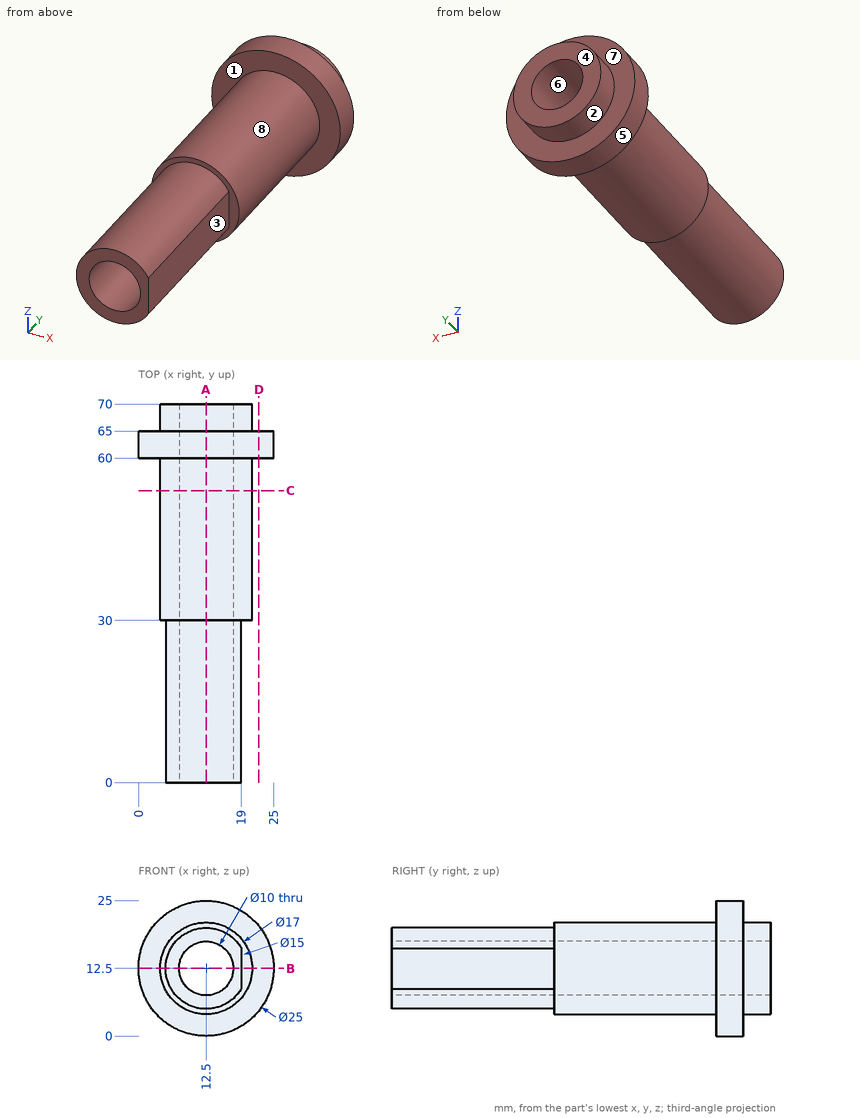
Here's the drawing with two shaded views (mm, measured from the low corner). I have some questions. A direction names the side the tool comes from. Coordinates: 2 decimals unless noted, no trailing zeros. Order: outer loops, then holes, each group sorted by start corner. A loop starts at its lowest first (then second) coordinate and runs counter-clockwise, first axis right, second up.
Item 1: I'm going to push flat-ended pins straight in: pin 1 Ø5 at (y, z) = (11.5, 7.5) entering from +X; pin 2 Ø8 at (x, y) = (21.5, 19.5) entering from -Z; pin 3 Ø1 at (x, y) = (7, 16) entering from +Z. Where does each tip first touch, or does it pass through?
Response values:
pin 1: stops at x = 19
pin 2: stops at z = 6.91
pin 3: stops at z = 18.09
Item 2: If we section it at B-B, the plane z = 12.5: List the corners of the cut face in (x, y) for me.
Response values:
outline: (0, 60) - (4, 60) - (4, 30) - (5, 30) - (5, 0) - (7.5, 0) - (7.5, 70) - (4, 70) - (4, 65) - (0, 65) - close; (17.5, 0) - (19, 0) - (19, 30) - (21, 30) - (21, 60) - (25, 60) - (25, 65) - (21, 65) - (21, 70) - (17.5, 70) - close
Item 3: If we section it at A-A, the plane x = 12.5: List the corners of the cut face in (y, z) for me.
Response values:
outline: (0, 5) - (30, 5) - (30, 4) - (60, 4) - (60, 0) - (65, 0) - (65, 4) - (70, 4) - (70, 7.5) - (0, 7.5) - close; (0, 17.5) - (70, 17.5) - (70, 21) - (65, 21) - (65, 25) - (60, 25) - (60, 21) - (30, 21) - (30, 20) - (0, 20) - close
Item 4: If we section it at C-C, the plane y = 54: List the corners of the cut face in (x, z) for me.
Response values:
outline: circle Ø17 at (12.5, 12.5); hole circle Ø10 at (12.5, 12.5)
Item 5: Which directions (+Z, -Z, +X, -X, +Y, -Y) give clear straight access to the entire face, cutting with the end or side of a thin tool? Please do the marked faces 1, 2, 3, 4 and 5.
Response values:
face 1: -Y
face 2: +Y
face 3: +Z, -Z, +X, -Y
face 4: +Z, -Z, +X, -X, +Y
face 5: +Y, -Y
Item 6: If we section it at D-D, the plane x = 22.25: List the corners of the cut face in (y, z) for me, then the cut area to 3 significant figures.
Response values:
outline: (60, 4.68) - (65, 4.68) - (65, 20.32) - (60, 20.32) - close
area: 78.2 mm2
Item 7: I need wall thicknesses on probe 1 along X at (y, z) = (20.5, 12.5); probe 2 along X at (y, z) = (48, 12.5); probe 3 along Z at (x, y) = (12.5, 21.5). Which ranges of each line are inside material? Lowest first, please.
Response values:
probe 1: x = 5 to 7.5, 17.5 to 19
probe 2: x = 4 to 7.5, 17.5 to 21
probe 3: z = 5 to 7.5, 17.5 to 20
Item 8: Thinking about a two-plate mould opening in Z: for the marked faces 6, 7 and 8, which applies, pulls with the +Z half, pulls with the -Z half, needs draft (parallel to the pull), parting line crosses it, or undercut?
Response values:
face 6: undercut
face 7: needs draft
face 8: parting line crosses it
